Study the drawing (mm; zero at the part's minimum x, y, z) and answer. A direction names the side the tool comes from. Give positions to 0.01 mm unless a question says otherwise; leave off trailing zeros. Write each loop counter-clockwise with the first axis right and the second up, starting at its lowest first coordinate (ties: lowest second). Pieces come first, ordered by that corner, then holes. Notation, with made-up numbers: (-1.75, 53.5) - (48.25, 53.5) arc R14 ccw to (48.25, 57.5) - close; hole circle Ø9 at (0, 8). An arc over 180 degrees is marked (long way). Answer in a Markdown table with one row per item. Add a question column.
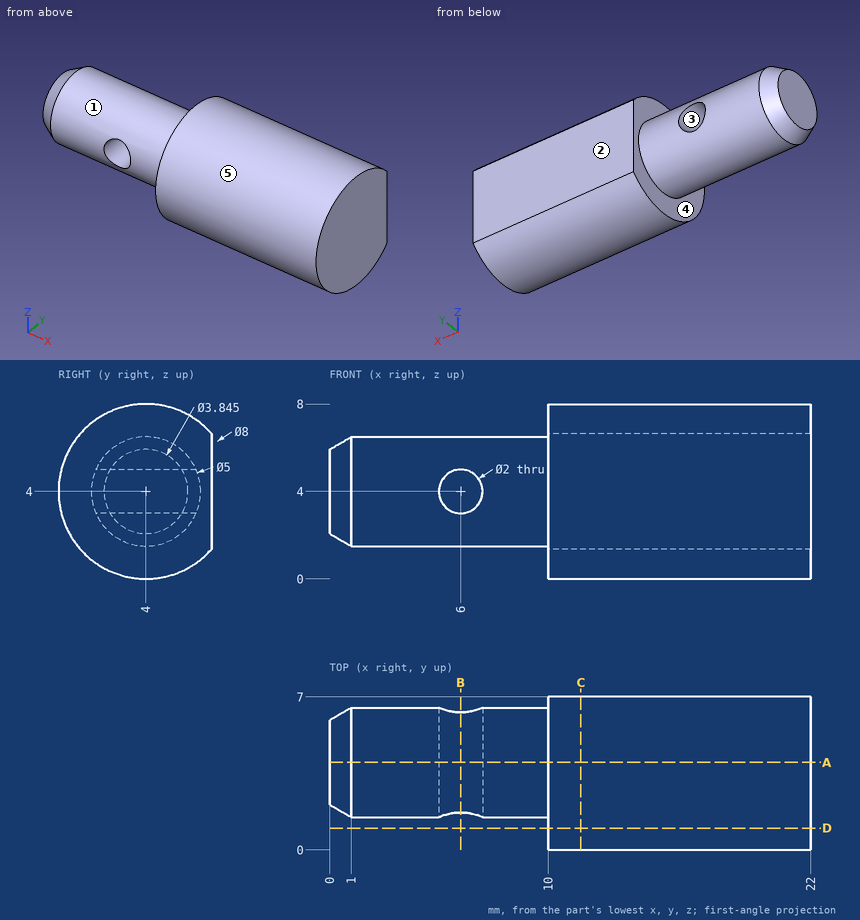
1. The mould has two halves that part along Z. Classify the marked faces 1, 2 and 3: +Z half, -Z half, draft (parallel to the pull), parting line (faces both ways), or undercut.
2. A tool of negligible diameter and unlimited length cuts with its end or side. For the marked faces 4 and 5, from which of +Z, -Z, +X, -X, +Y, -Y can it reach the whole face along a straight path? Write none if from no direction.
3. Section C-C (x = 11.5) is taken. Give the vertices of the cut face in (y, z).
4. Given pin 1 Ø3 at (x, y) = (4.5, 1) entering from +Z; pin 2 Ø2.5 at (x, z) = (6, 4) entering from +Y; pin 3 Ø1.5 at (x, z) = (4, 6) entering from +Y (1 decimal), each flat-ended and moving along its own axis, determine where each tip first touches the part or whether it passes through.
5. Section A-A (y = 4) is taken. Give the vertices of the cut face in (x, z).
6. Straight lines are drawn through the part: L1, parallel to X at y = 4.45, z = 4; L2, parallel to Y at x = 15, z = 7 (1 decimal); L3, parallel to Y at x = 2.25, z = 4. For each, find the intervals that lie inside material, in ascending order. Write a range as [from, to].
7. Section B-B (x = 6) is taken. Give the vertices of the cut face in (y, z).
8. Section D-D (y = 1) is taken. Give the vertices of the cut face in (x, z).
Geometry check:
| question | item | result |
|---|---|---|
| 1 | face 1 | parting line |
| 1 | face 2 | draft |
| 1 | face 3 | undercut |
| 2 | face 4 | -X |
| 2 | face 5 | +X, -X |
| 3 | outline | (7, 1.35) - (7, 6.65) arc R4 ccw (long way) to start |
| 4 | pin 1 | z = 6 |
| 4 | pin 2 | y = 6.5 |
| 4 | pin 3 | y = 6.2 |
| 5 | outline | (0, 2.08) - (1, 1.5) - (10, 1.5) - (10, 0) - (22, 0) - (22, 8) - (10, 8) - (10, 6.5) - (1, 6.5) - (0, 5.92) - close; hole circle Ø2 at (6, 4) |
| 6 | L1 | [0, 5], [7, 22] |
| 6 | L2 | [1.4, 6.6] |
| 6 | L3 | [1.5, 6.5] |
| 7 | outline | (1.71, 3) arc R2.5 ccw to (6.29, 3) - close; (1.71, 5) - (6.29, 5) arc R2.5 ccw to start |
| 8 | outline | (10, 1.35) - (22, 1.35) - (22, 6.65) - (10, 6.65) - close |
